Design review of the part built by this model. Coordinates are the model's own, in mm. A direction names the side the tool comes from. Coordinates: 2 decimals unless noted, no trailing zeros. Loops run counter-clockwise (first coordinate to the right, second up) from the corner with the lowest first, then second, coordinate; pieces in that order, holes last. Notation, with made-up numbers: M -12.5,56.25 L 3.5,56.25 A33 cw 3.5,92.25 Z; hole C 43,6.5 d6. An arc over 180 degrees is marked long. Answer as CSV lines item,"result". Start each with the question number.
Autodesk Inventor part; units mm, degrees
ref_plane "YZ Plane" through (0, 0, 0) normal (1, 0, 0) x (0, 1, 0)
ref_plane "XZ Plane" through (0, 0, 0) normal (0, 1, 0) x (-1, 0, 0)
ref_plane "XY Plane" through (0, 0, 0) normal (0, 0, 1) x (1, 0, 0)
sketch "スケッチ1" plane through (0, 0, 0) normal (0, 1, 0) x (-1, 0, 0)
  line L0 (-6, -6) -> (6, -6)
  line L1 (6, -6) -> (6, 6)
  line L2 (6, 6) -> (-6, 6)
  line L3 (-6, 6) -> (-6, -6)
  line L4 (-6, -6) -> (6, 6) construction
  line L5 (6, -6) -> (-6, 6) construction
  point P0 (0, 0)
  dimension "d0" = 12
extrude "押し出し1" add sketch "スケッチ1" along normal blind 7
fillet "フィレット1" radius 3 4 edges at (6, 3.5, 6) (6, 3.5, -6) (-6, 3.5, 6) (-6, 3.5, -6)
sketch "スケッチ2" plane through (0, 7, 0) normal (0, 1, 0) x (1, 0, 0)
  circle A0 centre (0, 0) radius 5
  circle A1 centre (-3.5355, 3.5355) radius 1.5
  circle A2 centre (3.5355, 3.5355) radius 1.5
  circle A3 centre (3.5355, -3.5355) radius 1.5
  circle A4 centre (-3.5355, -3.5355) radius 1.5
  line L0 (-3.5355, -3.5355) -> (3.5355, 3.5355) construction
  line L1 (-3.5355, 3.5355) -> (3.5355, -3.5355) construction
  line L2 (-8.4, 0) -> (8.4, 0)
  circle A5 centre (0, 0) radius 5.25
  point P0 (0, 0)
  point P1 (4.6181, -2.4972)
  point P2 (4.6181, 2.4972)
  point P3 (2.4972, 4.6181)
  point P4 (-2.4972, 4.6181)
  point P5 (-4.6181, 2.4972)
  point P6 (-4.6181, -2.4972)
  point P7 (-2.4972, -4.6181)
  point P8 (2.4972, -4.6181)
  dimension "d4" = 10
  dimension "d5" = 3
  dimension "d6" = 3
  dimension "d7" = 3
  dimension "d8" = 3
  dimension "d9" = 45
  dimension "d10" = 10.5
extrude "押し出し2" cut sketch "スケッチ2" against normal blind 3 contours L2 A5 A3 A0 | A0 A2 A5 L2 | A0 A2 A5 | A3 A5 A0 | L2 A5 A1 A0 | A0 A4 A5 L2 | A0 A1 A5 A2 | A5 A2 | A3 A5 A4 A0 | A3 A5 | A1 A5 A0 | A0 A4 A5 | A1 A5 | A5 A4
fillet "フィレット2" radius 0.2 1 edges at (-5, 7, 0)
properties part number "smd_power_inductor" material "アルミニウム 6061"
Item 1: For faces 4 (the face through (-6, 3, 0)), 5 (the face through (4.62, 5.52, -4.57)), list the 3-axis set-ups (+Z, -Z, +X, -X, +Y, -Y) from which the entire face can be reached by the end or side of a thin tool; tool diameter is ignored.
Item 2: Add section C-C (x = 0). Give the boundary of the cut face in (y, z), plus the area to 3 significant figures.
Item 3: Mouldability with a two-part tool opening along X and no side actions: class faces 1 (the face through (5.1, 3.55, 5.14)), 2 (the face through (-5.25, 5.52, -0.04)), 3 (the face through (0, 0, 0)) as released by +X, released by -X, zero draft, split by the parting line, or undercut.
Item 4: Add section B-B (z = 0). Give the boundary of the cut face in (x, y).
Item 5: For pin 1 (1.5 mm diameter, centred on x = 4.5, y = 3.5, fed in from -Z), flat-tipped, find the tip position at first contact; note if it passes through.
Item 6: For line 1 along Z through (x, y) = (1, 6.25); line 2 along Z through (x, y) = (0.5, 5); line 3 along Y through (x, z) = (-4.75, -3.5), list the stretches that pass through material, from the lowest coordinate up. Write a range as from..to.
Item 7: Add section A-A (y = 3.5). Give the boundary of the cut face in (x, z), plus the area to 3 significant figures.
Response:
1,face 4,"+Z, -Z, -X, +Y, -Y"
1,face 5,"+Y"
2,outline,"M 0,-6 L 7,-6 L 7,-5.25 L 4,-5.25 L 4,-5 L 6.8,-5 A0.2 ccw 7,-4.8 L 7,4.8 A0.2 ccw 6.8,5 L 4,5 L 4,5.25 L 7,5.25 L 7,6 L 0,6 Z"
2,area,"82.5 mm²"
3,face 1,"released by +X"
3,face 2,"undercut"
3,face 3,"zero draft"
4,outline,"M -6,0 L 6,0 L 6,7 L 5.25,7 L 5.25,4 L 5,4 L 5,6.8 A0.2 ccw 4.8,7 L -4.8,7 A0.2 ccw -5,6.8 L -5,4 L -5.25,4 L -5.25,7 L -6,7 Z"
5,pin 1,"z = -5.9"
6,line 1,"-6..-5.15, -4.9..4.9, 5.15..6"
6,line 2,"-6..-5.23, -4.97..4.97, 5.23..6"
6,line 3,"0..4"
7,outline,"M -6,-3 A3 ccw -3,-6 L 3,-6 A3 ccw 6,-3 L 6,3 A3 ccw 3,6 L -3,6 A3 ccw -6,3 Z"
7,area,"136 mm²"
